Geometry: final body of the model. Coordinates: model frame, mm. A direction names the side the tool comes from. Coordinates: 2 decimals unless noted, no trailing zeros. Write each loop counter-clockwise with the first axis right and the second up, starting at its lowest first coordinate (ties: lowest second). Pieces come first, ordered by that corner, then holes. Notation, with made-up numbers: (80, 85) -> (100, 85) arc R22 ccw to (100, 94) -> close; hole circle Ø1 at (16.25, -25.5). An arc over 180 degrees is marked (long way). One line per item, written item: value.
```python
from build123d import *

# Parameters (mm, degrees)
F0_W     = 749.3
F0_H     = 736.6
F1_DEPTH = 165.1
F2_T     = -19.05
F3_W     = 711.2
F3_H     = 38.1
F4_DEPTH = 25.4
F5_W     = 711.2
F5_H     = 44.45
F6_DEPTH = 19.05


with BuildPart() as f1:
    # F0 (on Top) → F1 (new body)
    with BuildSketch(Plane.XY):
        with Locations((-17.17346, 171.873332)):
            Rectangle(F0_W, F0_H)
    extrude(amount=F1_DEPTH)

    # F2
    f2_openings = [f1.faces().sort_by_distance(p)[0] for p in [
        (-17.17346, 171.873332, 0),
    ]]
    offset(amount=F2_T, openings=f2_openings)

    # F3 (on face) → F4 (join)
    with BuildSketch(Plane.XZ.offset(-521.123332)):
        with Locations((-17.17346, 19.05)):
            Rectangle(F3_W, F3_H)
    extrude(amount=F4_DEPTH)

    # F5 (on face) → F6 (join)
    with BuildSketch(Plane(origin=(0, -177.376668, 0), x_dir=(-1, 0, 0), z_dir=(0, 1, 0))):
        with Locations((17.17346, 22.225)):
            Rectangle(F5_W, F5_H)
    extrude(amount=F6_DEPTH)


solid = f1.part
```
(1) Section C-C (x = -4.5). Return the cut outline in (y, z).
Responses:
outline: (-196.43, 0) -> (-158.33, 0) -> (-158.33, 44.45) -> (-177.38, 44.45) -> (-177.38, 146.05) -> (521.12, 146.05) -> (521.12, 38.1) -> (495.72, 38.1) -> (495.72, 0) -> (540.17, 0) -> (540.17, 165.1) -> (-196.43, 165.1) -> close
(2) Reachability of faces 1 (the flat face through (-22, -177.377, 95)), 2 (the flat face through (357.477, 167, 81)), 3 (the flat face through (-12, -158.327, 23)) from +Z, -Z, +X, -X, +Y, -Y: full face, straight path, thin tool, end or side. Return the list, or none.
Responses:
face 1: none
face 2: +Z, -Z, +X, +Y, -Y
face 3: -Z
(3) First-contact query: pin 1 (2 mm diameter, centred on x = 68, y = 452, fed in from -Z). Flat tip, straight axial feed; report the tip coordinate or a pass-through.
Responses:
pin 1: stops at z = 146.05
(4) Section A-A (z = 135). Return the cut outline in (x, y), then the cut area to 3 significant figures.
Responses:
outline: (-391.82, -196.43) -> (357.48, -196.43) -> (357.48, 540.17) -> (-391.82, 540.17) -> close; hole (-372.77, -177.38) -> (338.43, -177.38) -> (338.43, 521.12) -> (-372.77, 521.12) -> close
area: 55,200 mm2
(5) Section B-B (y = 260). Return the cut outline in (x, z).
Responses:
outline: (-391.82, 0) -> (-372.77, 0) -> (-372.77, 146.05) -> (338.43, 146.05) -> (338.43, 0) -> (357.48, 0) -> (357.48, 165.1) -> (-391.82, 165.1) -> close
(6) Pull-direction query (X, two-part tool) for faces 4 (the flat face through (-22, 177, 165.1)), 5 (the flat face through (-22, 177, 146.05)), 6 (the flat face through (-391.823, 167, 81)), 7 (the flat face through (-22, 495.723, 19)); classes: released by +X, released by -X, zero draft, split by the parting line, or undercut.
Responses:
face 4: zero draft
face 5: undercut
face 6: released by -X
face 7: undercut
(7) Line query: line 1 (Y direction, x = -354, z = 14); line 2 (Y direction, x = -287.5, z = 133); line 3 (X direction, y = 30.5, z = 76.5). Output: solid intervals per line, ascending. Write a range as [from, to].
Responses:
line 1: y = [-196.43, -158.33], [495.72, 540.17]
line 2: y = [-196.43, -177.38], [521.12, 540.17]
line 3: x = [-391.82, -372.77], [338.43, 357.48]
